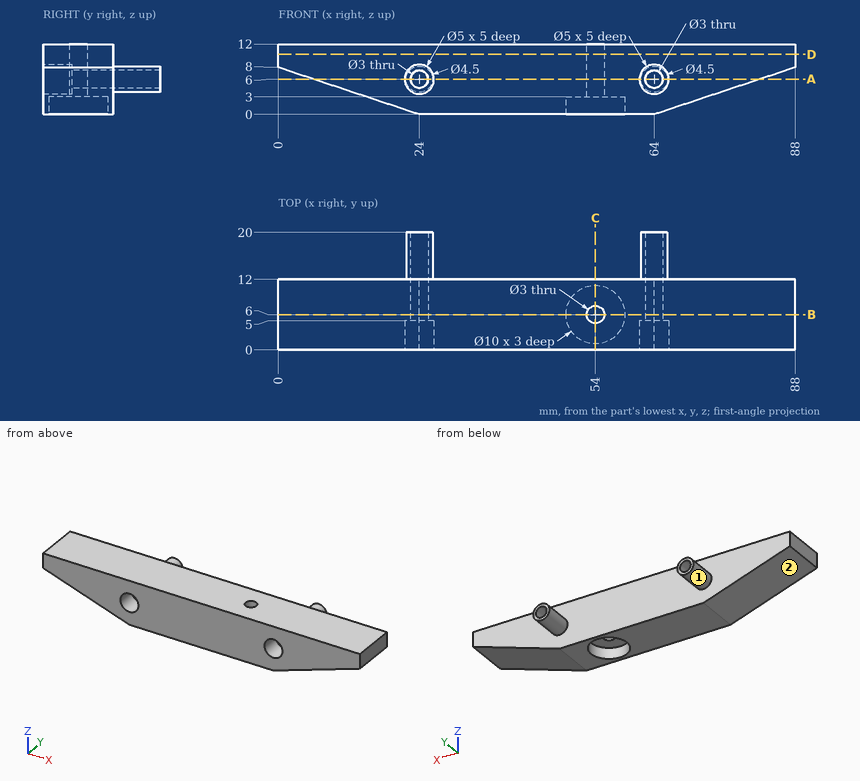
Input: dimensioned drawing with shaded views. Units: mm. Origin: part minimum x, y, z. A direction names the side the tool comes from. Round coordinates to 2 decimals unless told otherwise and drop trailing zeros. Order: outer loops, then holes, each group sorted by start corner. A loop starts at its lowest first (then second) coordinate and runs counter-clockwise, first axis right, second up. Notation, with made-up numbers: (65.5, 41.5) - (92.5, 41.5) arc R15 cw to (92.5, 63.5) - close; hole circle Ø6 at (84, 59.5). An arc over 180 degrees is marked (long way). Write item = value, one per line. Start each with the question number.
Q1. Pin query (flat end, axial travel): pin 1 (6 mm diameter, centred on x = 56, z = 8.5, fed in from +Y); pin 2 (4 mm diameter, centred on x = 54, z = 2, fed in from -Y); pin 3 (2.5 mm diameter, centred on x = 63.5, z = 5, fed in from -Y); pin 4 (8 mm diameter, centred on x = 54, y = 6, fed in from -Z). Return the tip coordinate at first contact, or that it passes through.
Q2. Ray query, line 1 (X direction, y = 12.75, z = 5); line 2 (Y direction, x = 60.5, z = 2.5); line 3 (Y direction, x = 53, z = 7). Return the intervals inside material, ascending. Write a range as from..to.
Q3. Cut plane D-D on z = 10.25. Return the cut outline in (x, y).
Q4. Cut plane B-B on y = 6. Return the cut outline in (x, z).
Q5. Access query for the marked faces 1 and 2. Directions: +Z, -Z, +X, -X, +Y, -Y. A direction counts if a zero-diameter tool reaches every point of the face in a straight line with its end or side. Return the directions, or none.
Q6. Cut plane A-A on z = 6. Give the number of separate pieces and of enclosed holes in the cut face, and give its area (3 significant figures).
Q7. Cut plane C-C on x = 54. Return the cut outline in (y, z).
Outcome:
q1.pin_1 = 12
q1.pin_2 = 0
q1.pin_3 = 5
q1.pin_4 = 3
q2.line_1 = 21.98..22.88, 25.12..26.02, 61.98..62.88, 65.12..66.02
q2.line_2 = 0..12
q2.line_3 = 0..4.88, 7.12..12
q3.outline = (0, 0) - (88, 0) - (88, 12) - (0, 12) - close; hole circle Ø3 at (54, 6)
q4.outline = (0, 8) - (24, 0) - (49, 0) - (49, 3) - (52.5, 3) - (52.5, 12) - (0, 12) - close; (55.5, 3) - (59, 3) - (59, 0) - (64, 0) - (88, 8) - (88, 12) - (55.5, 12) - close; hole circle Ø3 at (24, 6); hole circle Ø3 at (64, 6)
q5.face_1 = +Y
q5.face_2 = -Z, -X, +Y, -Y
q6.separate_pieces = 3
q6.enclosed_holes = 1
q6.area = 837 mm^2
q7.outline = (0, 0) - (1, 0) - (1, 3) - (4.5, 3) - (4.5, 12) - (0, 12) - close; (7.5, 3) - (11, 3) - (11, 0) - (12, 0) - (12, 12) - (7.5, 12) - close
